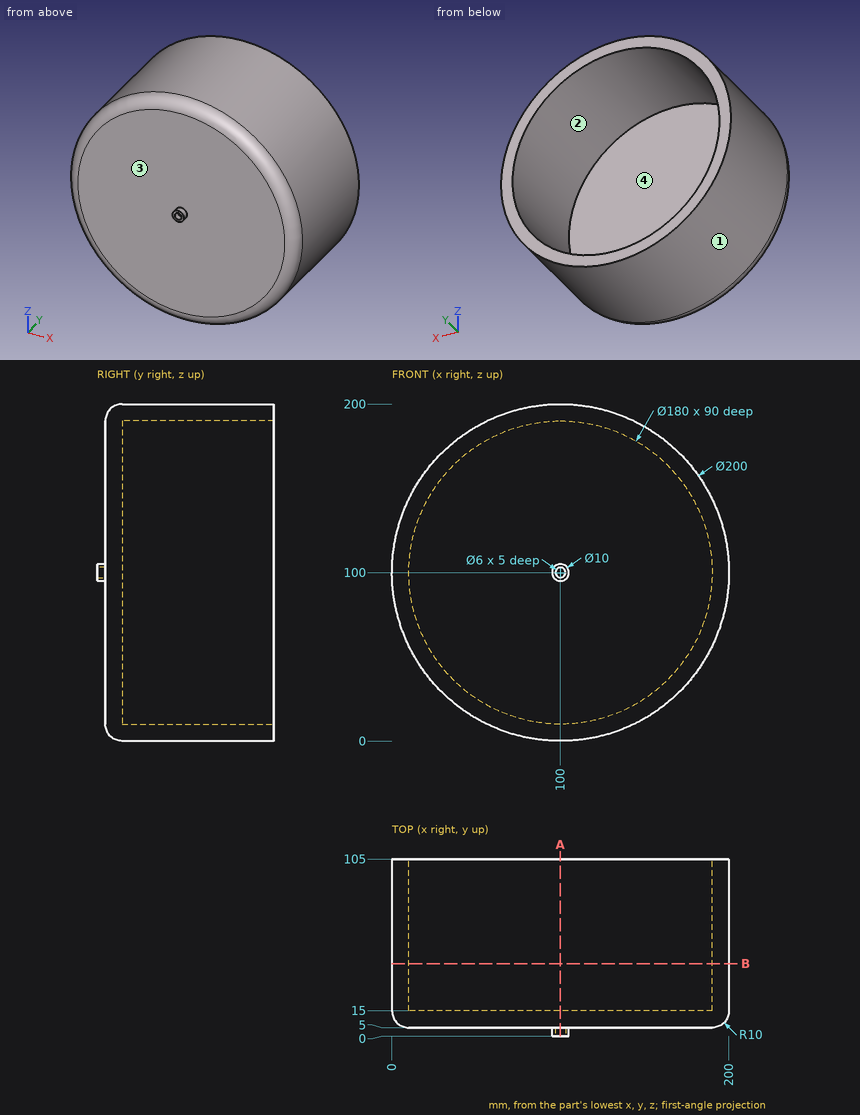
Here's the drawing with two shaded views (mm, measured from the low corner). I have some questions. Round coordinates to 2 decimals unless told otherwise and drop trailing zeros. Write each loop counter-clockwise with the first axis right and the second up, starting at its lowest first coordinate (ties: lowest second). Pieces come first, ordered by that corner, then holes. Notation, with made-up numbers: M -9.5,-5 L 40.5,-5 A10 ccw 40.5,11 Z; hole C -33.75,52.5 d6. An arc over 180 degrees is marked long. Answer in a Markdown table with one row per item. Add a question column.
Q1. Will these pins go through, and if not, where does the flat tip stop? pin 1 Ø2 at (x, y) = (105.5, 93.5) entering from +Z; pin 2 Ø3 at (x, z) = (99.5, 101) entering from -Y; pin 3 Ø4 at (y, z) = (14.5, 139.5) entering from +X.
Q2. If we mould it in two halves opening along X, with no side actions, what happens to the marked faces 1, 2, 3 and 4? For each: +X half, -X half, draft (parallel to the pull), parting line (faces both ways), or undercut.
Q3. If I drill on line 1 (X direction, y = 3.65, z = 100); line 2 (X direction, y = 58, z = 100); line 3 (Y direction, x = 104, z = 76), over which ranges is the centre line in solid material (lowest first)? Write a range as from..to.
Q4. Imagine slicing it at B-B (y = 43). Please give me the cut outline in (x, z), then the cut area to 3 significant figures.
Q5. Imagine slicing it at A-A (x = 100). Please give me the cut outline in (y, z), then the cut area to 3 significant figures.
Values:
| question | item | result |
|---|---|---|
| 1 | pin 1 | z = 199.9 |
| 1 | pin 2 | y = 5 |
| 1 | pin 3 | x = 192.69 |
| 2 | face 1 | parting line |
| 2 | face 2 | undercut |
| 2 | face 3 | draft |
| 2 | face 4 | undercut |
| 3 | line 1 | 95..97, 103..105 |
| 3 | line 2 | 0..10, 190..200 |
| 3 | line 3 | 5..15 |
| 4 | outline | C 100,100 d200; hole C 100,100 d180 |
| 4 | area | 5,970 mm^2 |
| 5 | outline | M 0,95 L 5,95 L 5,10 A10 ccw 15,0 L 105,0 L 105,10 L 15,10 L 15,190 L 105,190 L 105,200 L 15,200 A10 ccw 5,190 L 5,105 L 0,105 L 0,103 L 5,103 L 5,97 L 0,97 Z |
| 5 | area | 3,780 mm^2 |
